Geometry: final body of the model. Coordinates: model frame, mm. A direction names the side the tool comes from. Coordinates: 2 decimals unless noted, no trailing zeros. Loops run counter-clockwise (first coordinate to the right, second up) from the corner with the lowest first, then second, coordinate; pieces in that order, holes last. Notation, with made-up numbers: (64, 55.25) - (73, 55.25) arc R10 ccw to (73, 72.25) - close; hole circle Ø9 at (37, 56.25). An arc over 180 degrees is marked (long way). Put each result on its own line as item: value. Start each with the question number.
1) Section C-C on y = -25.5. Output: boundary loops of the cut face in (x, z), and give its area (3 significant figures).
2) Section D-D on z = -4.75. Output: boundary loops of the cut face in (x, y), and give its area (3 significant figures).
3) Reachability of faces 1 (the flat face through (9, 29.3, 0)), 2 (the flat face through (-34, -36, 0)), 3 (the flat face through (-34, 34, 0)), 4 (the flat face through (34, -36, 0)) from +Z, -Z, +X, -X, +Y, -Y: full face, straight path, thin tool, end or side. Return the list, or none.
4) Material intervals for line 1 along Y through (x, z) = (33, -1); line 2 along Y through (x, z) = (22, -9.5); line 3 along X through (y, z) = (-4, -1.75), sorted ascending. Write a range as from..to.
5) Section B-B on z = 1.5. Output: boundary loops of the cut face in (x, y).
6) Section A-A on x = -14. Output: boundary loops of the cut face in (y, z).
7) Contact query for flat-ended pins moving along their axis: pin 1 Ø3 at (y, z) = (-0.5, -3.5) entering from +X; pin 2 Ø6 at (x, z) = (-32, -6) entering from -Y; pin 3 Ø5.5 at (x, y) = (37.93, -37.93) entering from -Z; pin 4 Ø2 at (x, y) = (-37.93, 37.93) entering from -Z. Output: stop coordinate, or through.
8) Draft query along Y for faces 5 (the cylindrical face through (-36.312, -38.599, 1.521)), 6 (the flat face through (34, 34, 0)), 7 (the flat face through (-1, -45, 1)). Return one class per face: +Y half, -Y half, draft (parallel to the pull), parting line (faces both ways), or undercut.
```python
from build123d import *

# Parameters (mm, degrees)
SKETCH1_W           = 90
SKETCH1_H           = 90
BOSS_EXTRUDE1_DEPTH = 3
SKETCH9_R           = 45
SKETCH9_R_2         = 43
BOSS_EXTRUDE4_DEPTH = 10
SKETCH11_R          = 30.5
CUT_EXTRUDE9_DEPTH  = 58
SKETCH14_R          = 1.75
CUT_EXTRUDE10_DEPTH = 58


with BuildPart() as part:
    # Sketch1 → Boss-Extrude1 (new body)
    with BuildSketch(Plane.XY):
        Rectangle(SKETCH1_W, SKETCH1_H)
    extrude(amount=BOSS_EXTRUDE1_DEPTH)

    # Sketch9 → Boss-Extrude4 (add)
    with BuildSketch(Plane(origin=(0, 0, 0), x_dir=(-1, 0, 0), z_dir=(0, 0, -1))):
        Circle(SKETCH9_R)
        Circle(SKETCH9_R_2, mode=Mode.SUBTRACT)
    extrude(amount=BOSS_EXTRUDE4_DEPTH)

    # Sketch11 → Cut-Extrude9 (cut)
    with BuildSketch(Plane(origin=(0, 0, 0), x_dir=(-1, 0, 0), z_dir=(0, 0, -1))):
        Circle(SKETCH11_R)
    extrude(amount=-CUT_EXTRUDE9_DEPTH, mode=Mode.SUBTRACT)

    # Sketch14 → Cut-Extrude10 (cut)
    with BuildSketch(Plane.XY.offset(3)):
        with Locations((-37.928932188, 37.928932188)):
            Circle(SKETCH14_R)
        with Locations((37.928932188, 37.928932188)):
            Circle(SKETCH14_R)
        with Locations((37.928932188, -37.928932188)):
            Circle(SKETCH14_R)
        with Locations((-37.928932188, -37.928932188)):
            Circle(SKETCH14_R)
    extrude(amount=-CUT_EXTRUDE10_DEPTH, mode=Mode.SUBTRACT)


solid = part.part
```
Answer block:
1. outline: (-45, 0) - (-37.08, 0) - (-37.08, -10) - (-34.62, -10) - (-34.62, 0) - (-16.73, 0) - (-16.73, 3) - (-45, 3) - close; (16.73, 0) - (34.62, 0) - (34.62, -10) - (37.08, -10) - (37.08, 0) - (45, 0) - (45, 3) - (16.73, 3) - close
1. area: 219 mm²
2. outline: circle Ø90 at (0, 0); hole circle Ø86 at (0, 0)
2. area: 553 mm²
3. face 1: -Z
3. face 2: -Z, -X, -Y
3. face 3: -Z, -X, +Y
3. face 4: -Z, +X, -Y
4. line 1: y = -30.59..-27.57, 27.57..30.59
4. line 2: y = -39.26..-36.95, 36.95..39.26
4. line 3: x = -44.82..-42.81, 42.81..44.82
5. outline: (-45, -45) - (45, -45) - (45, 45) - (-45, 45) - close; hole circle Ø3.5 at (-37.93, -37.93); hole circle Ø3.5 at (-37.93, 37.93); hole circle Ø61 at (0, 0); hole circle Ø3.5 at (37.93, -37.93); hole circle Ø3.5 at (37.93, 37.93)
6. outline: (-45, 0) - (-42.77, 0) - (-42.77, -10) - (-40.66, -10) - (-40.66, 0) - (-27.1, 0) - (-27.1, 3) - (-45, 3) - close; (27.1, 0) - (40.66, 0) - (40.66, -10) - (42.77, -10) - (42.77, 0) - (45, 0) - (45, 3) - (27.1, 3) - close
7. pin 1: stops at x = 45
7. pin 2: stops at y = -34.41
7. pin 3: stops at z = 0
7. pin 4: passes through
8. face 5: undercut
8. face 6: draft
8. face 7: -Y half
